Input: part model. Units: mm. Frame: model coordinates. A direction names the side the tool comes from. Give positions to 0.01 mm unless a question says otherwise; leave off trailing zeros. Loops run counter-clockwise (first coordinate to the right, second up) from the corner with the lowest first, then second, coordinate; pieces in that order, holes last.
Autodesk Inventor part; units mm, degrees
ref_plane "Arbeitsebene2" through (-75, 27.1, 0) normal (0, 0, 1) x (0, 1, 0)
ref_plane "Arbeitsebene3" through (0, 99.4, -2.4) normal (-1, 0, 0) x (0, 0, 1)
ref_plane "Arbeitsebene1" through (-27.1, 0, 0) normal (1, 0, 0) x (0, 1, 0)
ref_plane "Arbeitsebene2" through (-75, 27.1, 0) normal (0, 0, 1) x (0, 1, 0)
sketch "center1" plane through (-75, 27.1, 0) normal (0, 0, 1) x (0, 1, 0)
  line L0 (-173.891, -75) -> (168.1592, -75)
  line L1 (0, 344.1359) -> (0, -385.7952)
  point P0 (-27.1, -75)
ref_plane "Arbeitsebene3" through (0, 99.4, -2.4) normal (-1, 0, 0) x (0, 0, 1)
sketch "center2" plane through (0, 99.4, -2.4) normal (-1, 0, 0) x (0, 0, 1)
  line L0 (184.8129, -72.3) -> (-258.9785, -72.3)
  point P0 (2.4, -99.4)
sketch "Groundplane" plane through (0, 0, 0) normal (0, 1, 0) x (-1, 0, 0)
  line L0 (45, 45) -> (-45, 45) construction
  line L1 (-45, 45) -> (-45, -45) construction
  line L2 (-45, -45) -> (45, -45) construction
  line L3 (45, -45) -> (45, 45) construction
  line L4 (1, 45) -> (-1, 45) construction
  line L5 (-1, 45) -> (-1, 40) construction
  line L6 (-1, 40) -> (1, 40) construction
  line L7 (1, 40) -> (1, 45) construction
  arc A0 (-1, 40) -> (1, 40) centre (0, 40) ccw construction
  line L8 (1, -45) -> (-1, -45) construction
  line L9 (-1, -45) -> (-1, -40) construction
  line L10 (-1, -40) -> (1, -40) construction
  line L11 (1, -40) -> (1, -45) construction
  arc A1 (1, -40) -> (-1, -40) centre (0, -40) ccw construction
  line L12 (0, -350.1368) -> (0, 271.1712)
  point P0 (0, 0)
  point P1 (0, -45)
  dimension "d5" = 2
  dimension "d6" = 5
  dimension "d7" = 2
  dimension "d8" = 5
  dimension "d9" = 90
  dimension "d63" = 90
  dimension "d76" = 45
sketch "Hallsensor" plane through (0, 0, 0) normal (1, 0, 0) x (0, 1, 0)
  line L0 (22.1, 0) -> (32.1, 0) construction
  line L1 (32.1, 0) -> (32.1, 20) construction
  line L2 (32.1, 20) -> (22.1, 20) construction
  line L3 (22.1, 20) -> (22.1, 0) construction
  line L4 (27.1, 182.4129) -> (27.1, -261.3785) construction
  line L5 (-146.791, 0) -> (195.2592, 0) construction
  line L6 (31.1, 1) -> (33.1, 1)
  line L7 (33.1, 1) -> (33.1, -1)
  line L8 (33.1, -1) -> (31.1, -1)
  line L9 (31.1, -1) -> (31.1, 1)
  line L10 (31.1, 1) -> (33.1, -1) construction
  line L11 (33.1, 1) -> (31.1, -1) construction
  line L12 (21.1, 1) -> (23.1, 1)
  line L13 (23.1, 1) -> (23.1, -1)
  line L14 (23.1, -1) -> (21.1, -1)
  line L15 (21.1, -1) -> (21.1, 1)
  line L16 (21.1, 1) -> (23.1, -1) construction
  line L17 (23.1, 1) -> (21.1, -1) construction
  line L18 (31.1, 21) -> (33.1, 21)
  line L19 (33.1, 21) -> (33.1, 19)
  line L20 (33.1, 19) -> (31.1, 19)
  line L21 (31.1, 19) -> (31.1, 21)
  line L22 (31.1, 21) -> (33.1, 19) construction
  line L23 (33.1, 21) -> (31.1, 19) construction
  line L24 (21.1, 21) -> (23.1, 21)
  line L25 (23.1, 21) -> (23.1, 19)
  line L26 (23.1, 19) -> (21.1, 19)
  line L27 (21.1, 19) -> (21.1, 21)
  line L28 (21.1, 21) -> (23.1, 19) construction
  line L29 (23.1, 21) -> (21.1, 19) construction
  line L30 (36.1, 30) -> (18.1, 30) construction
  line L31 (18.1, 30) -> (18.1, -20) construction
  line L32 (18.1, -20) -> (36.1, -20) construction
  line L33 (36.1, -20) -> (36.1, 30) construction
  circle A0 centre (27.1, 30) radius 1.6
  circle A1 centre (36.1, -20) radius 1.6
  circle A2 centre (18.1, -20) radius 1.6
  point P0 (0, 0)
  dimension "d127" = 20
  dimension "d128" = 5
  dimension "d129" = 5
  dimension "d130" = 2
  dimension "d131" = 20
  dimension "d132" = 4
  dimension "d133" = 4
  dimension "d134" = 10
  dimension "d135" = 3.2
ref_plane "Arbeitsebene1" through (-27.1, 0, 0) normal (1, 0, 0) x (0, 1, 0)
sketch "Montagepunkte" plane through (-27.1, 0, 0) normal (1, 0, 0) x (0, 1, 0)
  line L0 (27.1, 10) -> (27.1, -45.0561) construction
  line L1 (46.1, -45) -> (0, -45)
  line L2 (0, -45) -> (0, 35)
  line L3 (0, 35) -> (46.1, 35)
  line L4 (46.1, 35) -> (46.1, -45)
  circle A0 centre (36.1, -20) radius 1.6
  circle A1 centre (18.1, -20) radius 1.6
  circle A2 centre (27.1, 30) radius 1.6
  line L5 (36.1, -20) -> (18.1, -20) construction
  line L6 (18.1, -20) -> (18.1, -40) construction
  line L7 (18.1, -40) -> (36.1, -40) construction
  line L8 (36.1, -40) -> (36.1, -20) construction
  line L9 (27.1, 30) -> (27.1, 10) construction
  circle A3 centre (27.1, 10) radius 1.6
  circle A4 centre (36.1, -40) radius 1.6
  circle A5 centre (18.1, -40) radius 1.6
  point P0 (0, 0)
  point P1 (0, 0)
  point P2 (1.45, 0)
  dimension "d136" = 20
  dimension "d137" = 20
  dimension "d138" = 3.2
  dimension "d139" = 5
  dimension "d140" = 5
  dimension "d141" = 10
sketch "Skizze10" plane through (-27.1, 0, 0) normal (1, 0, 0) x (0, 1, 0)
  line L0 (46.1, -45) -> (0, -45)
  line L1 (0, -45) -> (0, 35)
  line L2 (0, 35) -> (46.1, 35)
  line L3 (46.1, 35) -> (46.1, -45)
  point P0 (0, 0)
extrude "Extrusion5" add sketch "Skizze10" along normal blind 5
sketch "Skizze11" plane through (-22.1, 0, 0) normal (1, 0, 0) x (0, 0, -1)
  line L0 (-35, 0) -> (45, 0)
  circle A0 centre (40, 36.1) radius 1.6
  circle A1 centre (20, 36.1) radius 1.6
  circle A2 centre (20, 18.1) radius 1.6
  circle A3 centre (40, 18.1) radius 1.6
  circle A4 centre (-10, 27.1) radius 1.6
  circle A5 centre (-30, 27.1) radius 1.6
  line L1 (-35, 32.1) -> (-5, 32.1)
  line L2 (-5, 32.1) -> (-5, 0)
  line L3 (-5, 0) -> (-35, 0)
  line L4 (-35, 0) -> (-35, 32.1)
  line L5 (15, 41.1) -> (45, 41.1)
  line L6 (45, 41.1) -> (45, 0)
  line L7 (45, 0) -> (15, 0)
  line L8 (15, 0) -> (15, 41.1)
  point P0 (0, 0)
  dimension "d142" = 5
  dimension "d143" = 5
  dimension "d144" = 5
  dimension "d145" = 5
  dimension "d146" = 5
  dimension "d147" = 5
extrude "Extrusion6" add sketch "Skizze11" along normal blind 3
chamfer "Fase3" distance 1 distance2 3 4 edges at (-19.1, 36.1, -18.4) (-19.1, 36.1, -38.4) (-19.1, 18.1, -38.4) (-19.1, 18.1, -18.4) measured on face at (-19.1, 5.5944, -26.9696)
chamfer "Fase4" distance 1 distance2 3 2 edges at (-19.1, 27.1, 31.6) (-19.1, 27.1, 11.6) measured on face at (-19.1, 8.5944, 16.9696)
sketch "Skizze12" plane through (0, 0, 0) normal (0, 1, 0) x (-1, 0, 0)
  line L0 (-45, 45) -> (-45, -45) construction
  line L1 (-45, -45) -> (45, -45) construction
  line L2 (45, -45) -> (45, 45) construction
  line L3 (45, 45) -> (-45, 45) construction
  arc A0 (1, -40) -> (-1, -40) centre (0, -40) ccw construction
  arc A1 (-1, 40) -> (1, 40) centre (0, 40) ccw construction
  circle A2 centre (0, 40) radius 1
  circle A3 centre (0, -40) radius 1
  line L4 (45, -45) -> (-45, -45)
  line L5 (-45, -45) -> (-45, 45)
  line L6 (-45, 45) -> (45, 45)
  line L7 (45, 45) -> (45, -45)
  point P0 (0, 0)
extrude "Extrusion7" add sketch "Skizze12" along normal blind 5
sketch "Skizze13" plane through (-27.1, 46.1, 35) normal (0, 0, 1) x (1, 0, 0)
  line L0 (0, -21.1) -> (-17.9, -41.1)
  line L1 (-17.9, -41.1) -> (0, -41.1)
  line L2 (0, -41.1) -> (0, -21.1)
  point P0 (27.1, -46.1)
  dimension "d108" = 20
extrude "Extrusion8" add sketch "Skizze13" against normal blind 5
sketch "Skizze14" plane through (-19.1, 46.1, -45) normal (0, 0, -1) x (-1, 0, 0)
  line L0 (25.9, -41.1) -> (8, -41.1)
  line L1 (25.9, -41.1) -> (8, -21.1)
  line L2 (8, -41.1) -> (8, -21.1)
  point P0 (-19.1, -46.1)
extrude "Extrusion9" add sketch "Skizze14" against normal blind 5
sketch "Skizze15" plane through (-27.1, 0, 0) normal (-1, 0, 0) x (0, 0, 1)
  line L0 (-12, 5) -> (3, 5)
  line L1 (3, 5) -> (3, 23)
  line L2 (-4, 30) -> (-5, 30)
  line L3 (-12, 23) -> (-12, 5)
  line L4 (-45, 5) -> (35, 5)
  arc A0 (-5, 30) -> (-12, 23) centre (-5, 23) ccw
  arc A1 (3, 23) -> (-4, 30) centre (-4, 23) ccw
  point P0 (0, 0)
  point P1 (3, 30)
  point P2 (-12, 30)
  point P3 (-40, 5)
  point P4 (30, 5)
  dimension "d114" = 15
  dimension "d115" = 25
  dimension "d116" = 7
extrude "Extrusion10" cut sketch "Skizze15" against normal through all
sketch "Skizze16" plane through (0, 5, 0) normal (0, 1, 0) x (1, 0, 0)
  line L0 (-9.1, 35) -> (35, 35)
  line L1 (35, 35) -> (35, -35)
  line L2 (35, -35) -> (-9.1, -35)
  line L3 (-9.1, -35) -> (-9.1, 35)
  line L4 (45, 45) -> (-19.1, 45)
  line L5 (45, -45) -> (45, 45)
  line L6 (-45, -45) -> (45, -45)
  line L7 (-19.1, -35) -> (-19.1, -5) construction
  point P0 (0, 0)
  dimension "d119" = 10
  dimension "d120" = 10
  dimension "d121" = 10
  dimension "d148" = 10
extrude "Extrusion11" cut sketch "Skizze16" against normal through all
sketch "Skizze17" plane through (-45, 0, 45) normal (0, -1, 0) x (1, 0, 0)
  line L0 (35.9, -80) -> (35.9, -10) construction
  line L1 (83, -45) -> (73, -51.0852)
  line L2 (73, -51.0852) -> (73, -47.2557)
  line L3 (73, -47.2557) -> (53, -47.2557)
  line L4 (53, -47.2557) -> (53, -41.9148)
  line L5 (53, -41.9148) -> (73, -41.9148)
  line L6 (73, -41.9148) -> (73, -38.0852)
  line L7 (73, -38.0852) -> (83, -45)
  line L8 (-520.1221, -45) -> (501.7814, -45)
  line L9 (35.9, -38.7956) -> (35.9, -51.0201)
  line L10 (35.9, -51.0201) -> (38.0698, -51.0201)
  line L11 (38.0698, -51.0201) -> (51.3295, -41.6603)
  line L12 (51.3295, -41.6603) -> (51.3295, -50.5946)
  line L13 (51.3295, -50.5946) -> (53.4, -50.5946)
  line L14 (53.4, -50.5946) -> (53.4, -39.0367)
  line L15 (53.4, -39.0367) -> (51.3011, -39.0367)
  line L16 (51.3011, -39.0367) -> (37.9705, -48.4957)
  line L17 (37.9705, -48.4957) -> (37.9705, -38.7956)
  line L18 (37.9705, -38.7956) -> (35.9, -38.7956)
  point P0 (45, -45)
extrude "Extrusion12" add sketch "Skizze17" against normal up to surface (5 mm away) contours L8 L14 L5 L6 L7 | L1 L2 L3 L14 L8 | L14 L3 L4 L8 | L8 L4 L5 L14 | L8 L12 L11 L16 L15 L14 L5 L4 | L4 L3 L14 L13 L12 L8 | L11 L10 L9 L8 L17 L16 | L8 L9 L18 L17
properties part number "HallSensor_Halterung"
(1) Mould query, pull axis Z, two halves, no side actions, for faces 5 (the flat face through (-19.1, 23, -30)), 6 (the flat face through (35, 3, -19)). Classes: +Z half, -Z half, draft (parallel to the pull), parting line (faces both ways), or undercut.
Values follow:
face 5: draft
face 6: undercut
(2) Cut plane B-B (z = 19). Return the cut outline in (x, y), and give its area (3 significant figures).
Values follow:
outline: (-45, 0) - (-9.1, 0) - (-9.1, 5) - (-19.1, 5) - (-19.1, 32.1) - (-22.1, 32.1) - (-22.1, 46.1) - (-27.1, 46.1) - (-27.1, 5) - (-45, 5) - close; (35, 0) - (45, 0) - (45, 5) - (35, 5) - close
area: 516 mm2
(3) Reachability of faces 1 (the flat face through (-21, 19, 5)), 2 (the flat face through (8.4, 2, -4)), 3 (the conical face through (-21.25, 19.69, -41.01)), 4 (the flat face through (-25, 14, 3)) from +Z, -Z, +X, -X, +Y, -Y: full face, straight path, thin tool, end or side. Return the list, or none.
Values follow:
face 1: +X, +Y
face 2: +Y, -Y
face 3: +X
face 4: +X, -X
(4) Cut plane D-D (y = 7.5). Return the cut outline in (x, z).
Values follow:
outline: (-42.76, -45) - (-19.1, -45) - (-19.1, -15) - (-22.1, -15) - (-22.1, -12) - (-27.1, -12) - (-27.1, -40) - (-42.76, -40) - close; (-42.76, 30) - (-27.1, 30) - (-27.1, 3) - (-22.1, 3) - (-22.1, 5) - (-19.1, 5) - (-19.1, 35) - (-42.76, 35) - close
(5) Cut plane A-A (x = 23). Return the cut outline in (y, z).
Values follow:
outline: (0, -45) - (5, -45) - (5, -35) - (0, -35) - close; (0, -2.26) - (5, -2.26) - (5, 3.09) - (0, 3.09) - close; (0, 35) - (5, 35) - (5, 45) - (0, 45) - close
(6) Pin query (flat end, axial travel): pin 1 Ø8 at (y, z) = (22, 27.5) entering from +X; pin 2 Ø1.9 at (y, z) = (27.1, 10) entering from +X; pin 3 Ø4 at (x, y) = (-25.5, 14.5) entering from +Z; pin 4 Ø1.2 at (x, z) = (0, 40) entering from -Y. Return the tip coordinate at first contact, or that it passes through.
Values follow:
pin 1: stops at x = -19.1
pin 2: stops at x = -22.1
pin 3: stops at z = 35
pin 4: passes through
(7) Ray query, probe 1 along Y at (x, z) = (-22.05, -40); probe 2 along Y at (x, z) = (-22.05, 30); probe 3 along Z at (x, y) = (-22, 36). Return the intervals inside material, ascending.
Values follow:
probe 1: y = 0 to 16.48, 19.72 to 34.48, 37.72 to 41.1
probe 2: y = 0 to 25.48, 28.72 to 32.1
probe 3: z = -45 to -41.63, -38.37 to -21.63, -18.37 to -15
